Check sheet for the modelled part. Datum: model origin and axes. Units: mm. Round coordinates to 2 decimals unless told otherwise and drop trailing zeros. Order: outer loops, then holes, each group sorted by start corner. A loop starts at its lowest first (then second) coordinate and runs counter-clockwise, first axis right, second up. Notation, with made-up numbers: (69.25, 75) -> (94.25, 75) arc R18 cw to (94.25, 83) -> close; hole circle Ø2 at (46.5, -25). An arc over 180 degrees is marked (long way). Use CSV: the item, a comma, the result in double quotes.
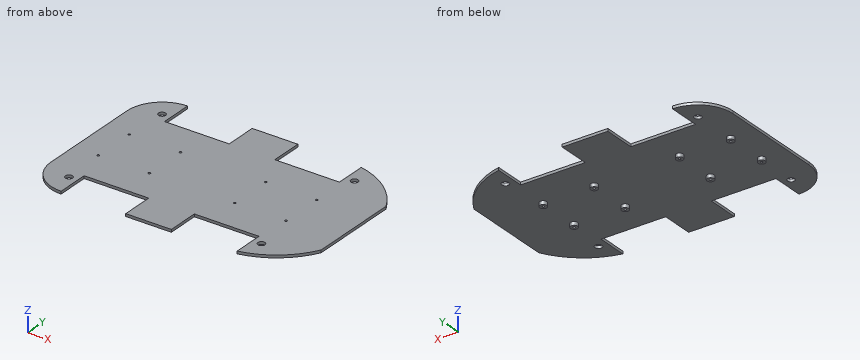
```python
from build123d import *

# Parameters (mm, degrees)
SKETCH_1_R          = 2
SKETCH_1_W          = 15
SKETCH_1_H          = 3
EXTRUDE_1_DEPTH     = 3
CUT_EXTRUDE_1_REACH = 360.482
SKETCH_2_W          = 15
SKETCH_2_H          = 3
SKETCH_3_R          = 2
EXTRUDE_2_DEPTH     = 3
SKETCH_4_W          = 15
SKETCH_4_H          = 3
CUT_EXTRUDE_2_DEPTH = 10
EXTRUDE_START       = -3
EXTRUDE_3_DEPTH     = 3
SKETCH_10_R         = 4
CUT_EXTRUDE_3_DEPTH = 3
SKETCH_11_R         = 1.35
CUT_EXTRUDE_4_DEPTH = 3
EXTRUDE_START_2     = 4
SKETCH_12_R         = 4
SKETCH_12_R_2       = 1.35
EXTRUDE_4_DEPTH     = 4
SKETCH_13_R         = 1.35
CUT_EXTRUDE_5_DEPTH = 3
SKETCH_14_R         = 4
SKETCH_14_R_2       = 1.35
EXTRUDE_5_DEPTH     = 4
CUT_EXTRUDE_START   = -4
CUT_EXTRUDE_6_DEPTH = 4


with BuildPart() as part:
    # 草图1 → 凸台-拉伸1 (new body)
    with BuildSketch(Plane.XY.offset(3)):
        with BuildLine():
            Line((165, 0), (165, 28))
            Line((165, 28), (173, 28))
            Line((173, 28), (173, 31.7))
            Line((173, 31.7), (188, 31.7))
            Line((188, 31.7), (188, 28))
            Line((188, 28), (238.3, 28))
            Line((238.3, 28), (238.3, 1.880138448))
            ThreePointArc((238.3, 1.880138448), (310, 90), (238.3, 178.119861552))
            Line((238.3, 178.119861552), (238.3, 152))
            Line((238.3, 152), (188, 152))
            Line((188, 152), (188, 148.3))
            Line((188, 148.3), (173, 148.3))
            Line((173, 148.3), (173, 152))
            Line((173, 152), (165, 152))
            Line((165, 152), (165, 180))
            Line((165, 180), (113.3, 180))
            Line((113.3, 180), (113.3, 152))
            Line((113.3, 152), (63, 152))
            Line((63, 152), (63, 148.3))
            Line((63, 148.3), (48, 148.3))
            Line((48, 148.3), (48, 152))
            Line((48, 152), (40, 152))
            Line((40, 152), (40, 180))
            ThreePointArc((40, 180), (11.715728753, 168.284271247), (0, 140))
            Line((0, 140), (0, 40))
            ThreePointArc((0, 40), (11.715728753, 11.715728753), (40, 0))
            Line((40, 0), (40, 28))
            Line((40, 28), (48, 28))
            Line((48, 28), (48, 31.7))
            Line((48, 31.7), (63, 31.7))
            Line((63, 31.7), (63, 28))
            Line((63, 28), (113.3, 28))
            Line((113.3, 28), (113.3, 0))
            Line((113.3, 0), (165, 0))
        make_face()
        with Locations(Location((233.9, 84.9, 0), (0, 0, 180))):
            Circle(SKETCH_1_R, mode=Mode.SUBTRACT)
        with Locations(Location((186.1, 84.9, 0), (0, 0, 180))):
            Circle(SKETCH_1_R, mode=Mode.SUBTRACT)
        with Locations(Location((28, 166, 0), (0, 0, 180))):
            Circle(SKETCH_1_R, mode=Mode.SUBTRACT)
        with Locations(Location((28, 14, 0), (0, 0, 180))):
            Circle(SKETCH_1_R, mode=Mode.SUBTRACT)
        with Locations(Location((248.3, 165.059930776, 0), (0, 0, 180))):
            Circle(SKETCH_1_R, mode=Mode.SUBTRACT)
        with Locations(Location((248.3, 14.940069224, 0), (0, 0, 180))):
            Circle(SKETCH_1_R, mode=Mode.SUBTRACT)
        with Locations(Location((139.15, 14, 0), (0, 0, 180))):
            Circle(SKETCH_1_R, mode=Mode.SUBTRACT)
        with Locations(Location((139.15, 166, 0), (0, 0, 180))):
            Circle(SKETCH_1_R, mode=Mode.SUBTRACT)
        with Locations((55.5, 52)):
            Rectangle(SKETCH_1_W, SKETCH_1_H, mode=Mode.SUBTRACT)
        with Locations((180.5, 52)):
            Rectangle(SKETCH_1_W, SKETCH_1_H, mode=Mode.SUBTRACT)
        with Locations((180.5, 128)):
            Rectangle(SKETCH_1_W, SKETCH_1_H, mode=Mode.SUBTRACT)
        with Locations((55.5, 128)):
            Rectangle(SKETCH_1_W, SKETCH_1_H, mode=Mode.SUBTRACT)
    extrude(amount=-EXTRUDE_1_DEPTH)

    # 草图2 → 切除-拉伸1 (cut, up to next)
    with BuildSketch(Plane(origin=(0, 0, 0), x_dir=(-1, 0, 0), z_dir=(0, 0, -1)), mode=Mode.PRIVATE) as cut_extrude_1_sk1:
        with Locations((-55.280073226, 119.6)):
            Rectangle(SKETCH_2_W, SKETCH_2_H)
    cut_extrude_1_tool1 = extrude(cut_extrude_1_sk1.sketch, amount=-CUT_EXTRUDE_1_REACH, mode=Mode.PRIVATE) & part.part
    # 草图2 → 切除-拉伸1 (cut, up to next)
    with BuildSketch(Plane(origin=(0, 0, 0), x_dir=(-1, 0, 0), z_dir=(0, 0, -1)), mode=Mode.PRIVATE) as cut_extrude_1_sk2:
        Polygon((-48, 152), (-40, 152), (-40, 143.6), (-48, 143.6), (-48, 139.9), (-63, 139.9), (-63, 143.6), (-113.3, 143.6), (-113.3, 152), (-63, 152), (-63, 148.3), (-48, 148.3), align=None)
    cut_extrude_1_tool2 = extrude(cut_extrude_1_sk2.sketch, amount=-CUT_EXTRUDE_1_REACH, mode=Mode.PRIVATE) & part.part
    add(cut_extrude_1_tool1.solids().sort_by_distance((55.280073, 119.6, 0))[0], mode=Mode.SUBTRACT)
    add(cut_extrude_1_tool2.solids().sort_by_distance((76.65, 147.042838, 0))[0], mode=Mode.SUBTRACT)

    # 草图3 → 凸台-拉伸2 (add)
    with BuildSketch(Plane.XY.offset(3)):
        with Locations((186.1, 84.9)):
            Circle(SKETCH_3_R)
        with Locations((233.9, 84.9)):
            Circle(SKETCH_3_R)
    extrude(amount=-EXTRUDE_2_DEPTH)

    # 草图4 → 切除-拉伸2 (cut)
    with BuildSketch(Plane(origin=(0, 0, 0), x_dir=(-1, 0, 0), z_dir=(0, 0, -1))):
        with Locations((-180.685567248, 119.6)):
            Rectangle(SKETCH_4_W, SKETCH_4_H)
        Polygon((-238.3, 143.6), (-188, 143.6), (-188, 139.9), (-173, 139.9), (-173, 143.6), (-165, 143.6), (-165, 152), (-173, 152), (-173, 148.3), (-188, 148.3), (-188, 152), (-238.3, 152), align=None)
    extrude(amount=-CUT_EXTRUDE_2_DEPTH, mode=Mode.SUBTRACT)

    # Split Bodies 4
    split(bisect_by=Plane.ZX.offset(90), keep=Keep.TOP)

    # 草图9 → 凸台-拉伸3 (add)
    with BuildSketch(Plane(origin=(0, 0, 0), x_dir=(-1, 0, 0), z_dir=(0, 0, -1)).offset(EXTRUDE_START)):
        with BuildLine():
            Line((-310, 80), (0, 80))
            Line((0, 80), (0, 140))
            ThreePointArc((0, 140), (-11.715728753, 168.284271247), (-40, 180))
            Line((-40, 180), (-40, 143.6))
            Line((-40, 143.6), (-113.3, 143.6))
            Line((-113.3, 143.6), (-113.3, 180))
            Line((-113.3, 180), (-165, 180))
            Line((-165, 180), (-165, 143.6))
            Line((-165, 143.6), (-238.3, 143.6))
            Line((-238.3, 143.6), (-238.3, 178.119861552))
            ThreePointArc((-238.3, 178.119861552), (-289.810457669, 146.802288686), (-310, 90))
            Line((-310, 90), (-310, 80))
        make_face()
    extrude(amount=EXTRUDE_3_DEPTH)

    # 草图10 → 切除-拉伸3 (cut)
    with BuildSketch(Plane(origin=(0, 0, 0), x_dir=(-1, 0, 0), z_dir=(0, 0, -1))):
        with Locations((-248.3, 153.6)):
            Circle(SKETCH_10_R)
        with Locations((-30, 153.6)):
            Circle(SKETCH_10_R)
    extrude(amount=-CUT_EXTRUDE_3_DEPTH, mode=Mode.SUBTRACT)

    # 镜向2: part across plane


with BuildPart() as part_1:
    add(part.part)
    add(part.part.mirror(Plane(origin=(310, 80, 328.729949498), x_dir=(0, 0, 1), z_dir=(0, -1, 0))))

    # 草图11 → 切除-拉伸4 (cut)
    with BuildSketch(Plane(origin=(0, 0, 0), x_dir=(-1, 0, 0), z_dir=(0, 0, -1))):
        with Locations((-86.022725282, 104.5)):
            Circle(SKETCH_11_R)
        with Locations((-86.022725282, 55.5)):
            Circle(SKETCH_11_R)
        with Locations((-28.022725282, 104.5)):
            Circle(SKETCH_11_R)
        with Locations((-28.022725282, 55.5)):
            Circle(SKETCH_11_R)
    extrude(amount=-CUT_EXTRUDE_4_DEPTH, mode=Mode.SUBTRACT)

    # 草图12 → 凸台-拉伸4 (add)
    # profile 1 of 4: a face of its own
    with BuildSketch(Plane(origin=(0, 0, 0), x_dir=(-1, 0, 0), z_dir=(0, 0, -1)).offset(EXTRUDE_START_2)):
        with Locations(Location((-86.022725282, 104.5, 0), (0, 0, 180))):
            Circle(SKETCH_12_R)
        with Locations((-86.022725282, 104.5)):
            Circle(SKETCH_12_R_2, mode=Mode.SUBTRACT)
    # profile 2 of 4: a face of its own
    with BuildSketch(Plane(origin=(0, 0, 0), x_dir=(-1, 0, 0), z_dir=(0, 0, -1)).offset(EXTRUDE_START_2)):
        with Locations(Location((-28.022725282, 104.5, 0), (0, 0, 180))):
            Circle(SKETCH_12_R)
        with Locations((-28.022725282, 104.5)):
            Circle(SKETCH_12_R_2, mode=Mode.SUBTRACT)
    # profile 3 of 4: a face of its own
    with BuildSketch(Plane(origin=(0, 0, 0), x_dir=(-1, 0, 0), z_dir=(0, 0, -1)).offset(EXTRUDE_START_2)):
        with Locations(Location((-28.022725282, 55.5, 0), (0, 0, 180))):
            Circle(SKETCH_12_R)
        with Locations((-28.022725282, 55.5)):
            Circle(SKETCH_12_R_2, mode=Mode.SUBTRACT)
    # profile 4 of 4: a face of its own
    with BuildSketch(Plane(origin=(0, 0, 0), x_dir=(-1, 0, 0), z_dir=(0, 0, -1)).offset(EXTRUDE_START_2)):
        with Locations(Location((-86.022725282, 55.5, 0), (0, 0, 180))):
            Circle(SKETCH_12_R)
        with Locations((-86.022725282, 55.5)):
            Circle(SKETCH_12_R_2, mode=Mode.SUBTRACT)
    extrude(amount=-EXTRUDE_4_DEPTH)

    # 草图13 → 切除-拉伸5 (cut)
    with BuildSketch(Plane(origin=(0, 0, 0), x_dir=(-1, 0, 0), z_dir=(0, 0, -1))):
        with Locations((-183.092928671, 55.103896104)):
            Circle(SKETCH_13_R)
        with Locations((-183.092928671, 104.103896104)):
            Circle(SKETCH_13_R)
        with Locations((-241.09213252, 103.8)):
            Circle(SKETCH_13_R)
        with Locations((-241.092928671, 55.103896104)):
            Circle(SKETCH_13_R)
    extrude(amount=-CUT_EXTRUDE_5_DEPTH, mode=Mode.SUBTRACT)

    # 草图14 → 凸台-拉伸5 (add)
    # profile 1 of 4: a face of its own
    with BuildSketch(Plane(origin=(0, 0, 0), x_dir=(-1, 0, 0), z_dir=(0, 0, -1)).offset(EXTRUDE_START_2)):
        with Locations(Location((-241.09213252, 103.8, 0), (0, 0, 180))):
            Circle(SKETCH_14_R)
        with Locations((-241.09213252, 103.8)):
            Circle(SKETCH_14_R_2, mode=Mode.SUBTRACT)
    # profile 2 of 4: a face of its own
    with BuildSketch(Plane(origin=(0, 0, 0), x_dir=(-1, 0, 0), z_dir=(0, 0, -1)).offset(EXTRUDE_START_2)):
        with Locations(Location((-183.092928671, 104.103896104, 0), (0, 0, 180))):
            Circle(SKETCH_14_R)
        with Locations((-183.092928671, 104.103896104)):
            Circle(SKETCH_14_R_2, mode=Mode.SUBTRACT)
    # profile 3 of 4: a face of its own
    with BuildSketch(Plane(origin=(0, 0, 0), x_dir=(-1, 0, 0), z_dir=(0, 0, -1)).offset(EXTRUDE_START_2)):
        with Locations(Location((-241.092928671, 55.103896104, 0), (0, 0, 180))):
            Circle(SKETCH_14_R)
        with Locations((-241.092928671, 55.103896104)):
            Circle(SKETCH_14_R_2, mode=Mode.SUBTRACT)
    # profile 4 of 4: a face of its own
    with BuildSketch(Plane(origin=(0, 0, 0), x_dir=(-1, 0, 0), z_dir=(0, 0, -1)).offset(EXTRUDE_START_2)):
        with Locations(Location((-183.092928671, 55.103896104, 0), (0, 0, 180))):
            Circle(SKETCH_14_R)
        with Locations((-183.092928671, 55.103896104)):
            Circle(SKETCH_14_R_2, mode=Mode.SUBTRACT)
    extrude(amount=-EXTRUDE_5_DEPTH)

    # 草图15 → 切除-拉伸6 (cut)
    with BuildSketch(Plane(origin=(0, 0, 0), x_dir=(-1, 0, 0), z_dir=(0, 0, -1)).offset(CUT_EXTRUDE_START)):
        with BuildLine():
            Line((-300, 131.231056256), (-300, 28.768943744))
            ThreePointArc((-300, 28.768943744), (-307.464278423, 48.786796564), (-310, 70))
            Line((-310, 70), (-310, 90))
            ThreePointArc((-310, 90), (-307.464278423, 111.213203436), (-300, 131.231056256))
        make_face()
    extrude(amount=CUT_EXTRUDE_6_DEPTH, mode=Mode.SUBTRACT)


solid = part_1.part
```
Q1. Sectioned sample at C-C, the plane y = 6.4. Enter the section's corners in (x, z), then the cut area to 3 significant figures.
Result sheet:
outline,"(2.38, 0) -> (26, 0) -> (26, 3) -> (2.38, 3) -> close; (34, 0) -> (40, 0) -> (40, 3) -> (34, 3) -> close; (113.3, 0) -> (165, 0) -> (165, 3) -> (113.3, 3) -> close; (238.3, 0) -> (244.3, 0) -> (244.3, 3) -> (238.3, 3) -> close; (252.3, 0) -> (283.68, 0) -> (283.68, 3) -> (252.3, 3) -> close"
area,"356 mm^2"
Q2. Sectioned sample at D-D, the plane x = 152.5. Enter the section's corners in (y, z).
Result sheet:
outline,"(-20, 0) -> (180, 0) -> (180, 3) -> (-20, 3) -> close"
Q3. Sectioned sample at B-B, the plane x = 248.3. Enter the section's corners in (y, z), then the cut area to 3 significant figures.
Result sheet:
outline,"(-15.43, 0) -> (2.4, 0) -> (2.4, 3) -> (-15.43, 3) -> close; (10.4, 0) -> (149.6, 0) -> (149.6, 3) -> (10.4, 3) -> close; (157.6, 0) -> (175.43, 0) -> (175.43, 3) -> (157.6, 3) -> close"
area,"525 mm^2"
Q4. Scan lines: L1, parallel to Y at x = 86, z = -1; L2, parallel to Y at x = 85, z = 0.5; L3, parallel to X at y = 106, z = -3.5. Record each from-to range of solid material in increasing order.
Result sheet:
L1,"y = 51.5 to 54.15, 56.85 to 59.5, 100.5 to 103.15, 105.85 to 108.5"
L2,"y = 16.4 to 54.62, 56.38 to 103.62, 105.38 to 143.6"
L3,"x = 24.31 to 31.73, 82.31 to 89.73, 179.57 to 186.61, 237.75 to 244.43"
Q5. Sectioned sample at A-A, the plane z = -2. State how many separate pieces and enclosed holes the cut face has, then the cut area to 3 significant figures.
Result sheet:
separate pieces,"8"
enclosed holes,"8"
area,"356 mm^2"
Q6. Go/stop test with flat-tipped pins: pin 1 (0.9 mm diameter, centred on x = 210, z = 1.5, fed in from +Y); pin 2 (3.5 mm diameter, centred on y = 154.5, z = 1, fed in from -X); pin 3 (1.5 mm diameter, centred on y = 1, z = 1, fed in from -X). Record where each tip stops, or that it passes through.
Result sheet:
pin 1,"stops at y = 143.6"
pin 2,"stops at x = 2.09"
pin 3,"stops at x = 4.41"
